Read the model definition and answer for the solid it produces. Units are mm, in the model's axes. Round coordinates to 2 decimals unless told otherwise and drop trailing zeros. Loops run counter-clockwise (first coordinate to the right, second up) from the corner with the lowest first, then second, coordinate; pieces in that order, holes last. Notation, with made-up numbers: M 47.5,43 L 96.5,43 A20 cw 96.5,76 Z; hole C 15.5,-36.5 d3. An arc over 180 degrees is marked long. Write each question's results on one line, items separated by ' | '.
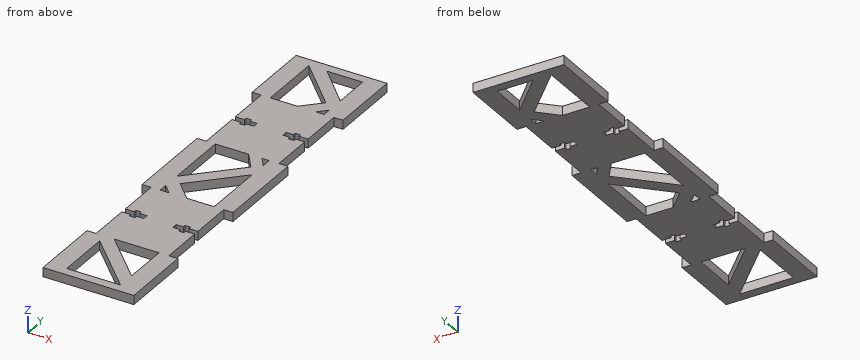
from build123d import *

# Parameters (mm, degrees)
SKETCH1_W           = 50
SKETCH1_H           = 230
BOSS_EXTRUDE1_DEPTH = 5
SKETCH9_W           = 5
SKETCH9_H           = 50
CUT_EXTRUDE6_DEPTH  = 7
SKETCH10_R          = 1.5
CUT_EXTRUDE7_DEPTH  = 7
CUT_EXTRUDE8_START  = -7
SKETCH11_R          = 1.5
CUT_EXTRUDE8_DEPTH  = 7
CUT_EXTRUDE9_DEPTH  = 7
SKETCH13_W          = 40
SKETCH13_H          = 50
BOSS_EXTRUDE2_DEPTH = 5
CUT_EXTRUDE10_DEPTH = 5


with BuildPart() as part:
    # Sketch1 → Boss-Extrude1 (new body)
    with BuildSketch(Plane.XY):
        Rectangle(SKETCH1_W, SKETCH1_H)
    extrude(amount=BOSS_EXTRUDE1_DEPTH)

    # Sketch9 → Cut-Extrude6 (cut)
    with BuildSketch(Plane.XY.offset(5)):
        with Locations((-22.5, 50)):
            Rectangle(SKETCH9_W, SKETCH9_H)
        with Locations((-22.5, -50)):
            Rectangle(SKETCH9_W, SKETCH9_H)
        with Locations((22.5, -50)):
            Rectangle(SKETCH9_W, SKETCH9_H)
        with Locations((22.5, 50)):
            Rectangle(SKETCH9_W, SKETCH9_H)
    extrude(amount=-CUT_EXTRUDE6_DEPTH, mode=Mode.SUBTRACT)

    # Sketch10 → Cut-Extrude7 (cut)
    with BuildSketch(Plane.ZY.offset(20)):
        with Locations(Location((2.5, 50, 0), (0, 0, 270))):
            Circle(SKETCH10_R)
        with Locations(Location((2.5, -50, 0), (0, 0, 270))):
            Circle(SKETCH10_R)
    extrude(amount=-CUT_EXTRUDE7_DEPTH, mode=Mode.SUBTRACT)

    # Sketch11 → Cut-Extrude8 (cut)
    with BuildSketch(Plane(origin=(20, 0, 0), x_dir=(0, 0, -1), z_dir=(1, 0, 0)).offset(CUT_EXTRUDE8_START)):
        with Locations(Location((-2.5, -50, 0), (0, 0, 270))):
            Circle(SKETCH11_R)
        with Locations(Location((-2.5, 50, 0), (0, 0, 270))):
            Circle(SKETCH11_R)
    extrude(amount=CUT_EXTRUDE8_DEPTH, mode=Mode.SUBTRACT)

    # Sketch12 → Cut-Extrude9 (cut)
    with BuildSketch(Plane.XY.offset(5)):
        Polygon((9.705882353, 84.705882353), (-15, 110), (-15, 60), align=None)
        Polygon((14.647058824, 19.647058824), (14.647058824, 79.647058824), (-10.764705882, 54.235294118), align=None)
        Polygon((10.411764706, 15.411764706), (-15, 50), (-15, -10), align=None)
        Polygon((14.647058824, 110), (-5, 110), (14.647058824, 89.647058824), align=None)
        Polygon((14.647058824, -40.352941176), (14.647058824, 9.647058824), (-10.058823529, -15.058823529), align=None)
        Polygon((9.705882353, -45.294117647), (-15, -20), (-15, -70), align=None)
        Polygon((14.647058824, -100), (14.647058824, -50.352941176), (-10.029585799, -75.029585799), align=None)
        Polygon((14.647058824, -110), (-15, -80), (-15, -110), align=None)
    extrude(amount=-CUT_EXTRUDE9_DEPTH, mode=Mode.SUBTRACT)

    # Sketch13 → Boss-Extrude2 (add)
    with BuildSketch(Plane.XY.offset(5)):
        with Locations((0, -50)):
            Rectangle(SKETCH13_W, SKETCH13_H)
        with Locations((0, 50)):
            Rectangle(SKETCH13_W, SKETCH13_H)
    extrude(amount=-BOSS_EXTRUDE2_DEPTH)

    # Sketch14 → Cut-Extrude10 (cut)
    with BuildSketch(Plane.XY.offset(5)):
        Polygon((-15, -48.5), (-15, -47), (-12, -47), (-12, -48.5), (-8, -48.5), (-8, -51.5), (-12, -51.5), (-12, -53), (-15, -53), (-15, -51.5), (-20, -51.5), (-20, -48.5), align=None)
        Polygon((-20, 48.5), (-15, 48.5), (-15, 47), (-12, 47), (-12, 48.5), (-8, 48.5), (-8, 51.5), (-12, 51.5), (-12, 53), (-15, 53), (-15, 51.5), (-20, 51.5), align=None)
        Polygon((15, -48.5), (15, -47), (12, -47), (12, -48.5), (8, -48.5), (8, -51.5), (12, -51.5), (12, -53), (15, -53), (15, -51.5), (20, -51.5), (20, -48.5), align=None)
        Polygon((20, 48.5), (15, 48.5), (15, 47), (12, 47), (12, 48.5), (8, 48.5), (8, 51.5), (12, 51.5), (12, 53), (15, 53), (15, 51.5), (20, 51.5), align=None)
    extrude(amount=-CUT_EXTRUDE10_DEPTH, mode=Mode.SUBTRACT)


solid = part.part
Item 1: The part is cut by section B-B (x = -17.5). Determine the outline of the cut face in (y, z), plus the area to 3 significant figures.
Outcome:
outline: M -115,0 L -51.5,0 L -51.5,5 L -115,5 Z; M -48.5,0 L 48.5,0 L 48.5,5 L -48.5,5 Z; M 51.5,0 L 115,0 L 115,5 L 51.5,5 Z | area: 1,120 mm2
Item 2: Straight lines are drawn through the part: line 1 (Y direction, x = 16, z = 0.85); line 2 (X direction, y = 23.5, z = 2.05); line 3 (X direction, y = -95.5, z = 2.85). For each, find the intervals that lie inside material, in ascending order.
Outcome:
line 1: y = -115 to -51.5, -48.5 to 48.5, 51.5 to 115 | line 2: x = -25 to -15, 4.47 to 11.82, 14.65 to 25 | line 3: x = -25 to -15, 0.32 to 10.2, 14.65 to 25
Item 3: The part is cut by section D-D (y = 38). Determine the outline of the cut face in (x, z).
Outcome:
outline: M -20,0 L 20,0 L 20,5 L -20,5 Z
Item 4: Flat-ended cylindrical pins translate along their axes: pin 1 (1.6 mm diameter, centred on y = 52.5, z = 2.5, fed in from +X); pin 2 (1.5 mm diameter, centred on y = -32, z = 1.5, fed in from -X). Find the tip coordinate at first contact, or state that the pin passes through.
Outcome:
pin 1: stops at x = 20 | pin 2: stops at x = -20
Item 5: The part is cut by section C-C (z = 3.1). State how many separate pieces and enclosed holes the cut face has, plus the area to 3 significant figures.
Outcome:
separate pieces: 1 | enclosed holes: 9 | area: 7,790 mm2
Item 6: The part is cut by section A-A (y = -7). Determine the outline of the cut face in (x, z).
Outcome:
outline: M -25,0 L -15,0 L -15,5 L -25,5 Z; M -12,0 L -2,0 L -2,5 L -12,5 Z; M 14.65,0 L 25,0 L 25,5 L 14.65,5 Z
